Autodesk Inventor part; units mm, degrees
ref_plane "YZ Plane" through (0, 0, 0) normal (1, 0, 0) x (0, 1, 0)
ref_plane "XZ Plane" through (0, 0, 0) normal (0, 1, 0) x (-1, 0, 0)
ref_plane "XY Plane" through (0, 0, 0) normal (0, 0, 1) x (1, 0, 0)
sketch "Sketch1" plane through (0, 0, 0) normal (0, 1, 0) x (-1, 0, 0)
  line L0 (-43.3, -50.05) -> (43.3, -50.05)
  line L1 (43.3, -50.05) -> (43.3, 50.05)
  line L2 (43.3, 50.05) -> (-43.3, 50.05)
  line L3 (-43.3, 50.05) -> (-43.3, -50.05)
  line L4 (-43.3, -50.05) -> (43.3, 50.05) construction
  line L5 (43.3, -50.05) -> (-43.3, 50.05) construction
  point P0 (0, 0)
  dimension "d0" = 86.6
  dimension "d1" = 100.1
extrude "Extrusion1" add sketch "Sketch1" along normal blind 4.445
sketch "Sketch2" plane through (0, 4.445, 0) normal (0, 1, 0) x (1, 0, 0)
  line L0 (40.1, 46.85) -> (-40.1, 46.85)
  line L1 (-40.1, 46.85) -> (-40.1, -46.85)
  line L2 (-40.1, -46.85) -> (40.1, -46.85)
  line L3 (40.1, -46.85) -> (40.1, 46.85)
  line L4 (40.1, 46.85) -> (-40.1, -46.85) construction
  line L5 (-40.1, 46.85) -> (40.1, -46.85) construction
  line L6 (-43.3, 50.05) -> (-43.3, -50.05)
  line L7 (-43.3, -50.05) -> (43.3, -50.05)
  line L8 (43.3, 50.05) -> (-43.3, 50.05)
  line L9 (43.3, -50.05) -> (43.3, 50.05)
  line L10 (36.9, -43.65) -> (43.3, -50.05) construction
  line L11 (34.4431, -46.85) -> (40.4716, -52.8784)
  line L12 (46.1284, -47.2216) -> (40.1, -41.1931)
  arc A0 (40.4716, -52.8784) -> (46.1284, -47.2216) centre (43.3, -50.05) ccw
  circle A1 centre (43.3, -50.05) radius 1.375
  point P0 (0, 0)
  dimension "d4" = 3.2
  dimension "d5" = 3.2
  dimension "d22" = 8
  dimension "d23" = 2.75
extrude "Extrusion2" add sketch "Sketch2" along normal blind 49 contours L0 L1 L2 L11 L7 L6 L8 L9 L12 L3 | L12 L9 A1 L7 L11 L2 L3 | L9 L7 A1 picked at (42.4402, -49.7491)
sketch "Sketch4" plane through (0, 0, 0) normal (0, -1, 0) x (1, 0, 0)
  line L0 (41.7906, 48.7379) -> (44.8094, 51.3621) construction
  line L1 (43.3, 50.05) -> (43.3, -50.05)
  line L2 (43.3, 44.7499) -> (47.4337, 48.3433)
  line L3 (42.1852, 54.381) -> (39.1663, 51.7567)
  arc A0 (39.1663, 51.7567) -> (38.0119, 50.05) centre (41.7906, 48.7379) ccw
  arc A1 (47.4337, 48.3433) -> (42.1852, 54.381) centre (44.8094, 51.3621) ccw
  line L4 (-43.3, 50.05) -> (43.3, 50.05)
  line L5 (38.0119, 50.05) -> (43.3, 50.05)
  line L6 (43.3, 50.05) -> (43.3, 44.7499)
  circle A2 centre (44.8094, 51.3621) radius 1.985
  line L7 (0, 50.05) -> (0, -50.05) construction
  line L8 (43.3, -50.05) -> (-43.3, -50.05) construction
  line L9 (43.3, 0) -> (-33.3, 0) construction
  line L10 (43.3, -50.05) -> (43.3, 50.05)
  line L11 (43.3, -44.7499) -> (47.4337, -48.3433)
  line L12 (42.1852, -54.381) -> (39.1663, -51.7567)
  arc A3 (38.0119, -50.05) -> (39.1663, -51.7567) centre (41.7906, -48.7379) ccw
  arc A4 (42.1852, -54.381) -> (47.4337, -48.3433) centre (44.8094, -51.3621) ccw
  line L13 (-43.3, -50.05) -> (43.3, -50.05)
  circle A5 centre (44.8094, -51.3621) radius 1.985
  line L14 (-43.3, 50.05) -> (-43.3, -50.05)
  line L15 (-43.3, 44.7499) -> (-47.4337, 48.3433)
  line L16 (-42.1852, 54.381) -> (-39.1663, 51.7567)
  arc A6 (-38.0119, 50.05) -> (-39.1663, 51.7567) centre (-41.7906, 48.7379) ccw
  arc A7 (-42.1852, 54.381) -> (-47.4337, 48.3433) centre (-44.8094, 51.3621) ccw
  line L17 (-38.0119, 50.05) -> (-43.3, 50.05)
  circle A8 centre (-44.8094, 51.3621) radius 1.985
  arc A9 (-47.4337, -48.3433) -> (-42.1852, -54.381) centre (-44.8094, -51.3621) ccw
  line L18 (-43.3, -44.7499) -> (-47.4337, -48.3433)
  line L19 (-42.1852, -54.381) -> (-39.1663, -51.7567)
  arc A10 (-39.1663, -51.7567) -> (-38.0119, -50.05) centre (-41.7906, -48.7379) ccw
  circle A11 centre (-44.8094, -51.3621) radius 1.985
  line L20 (-38.0119, -50.05) -> (-43.3, -50.05)
  line L21 (-43.3, -50.05) -> (-43.3, 50.05)
  point P0 (0, 0)
  point P1 (-38.0119, -50.05)
  point P2 (-43.3, -44.7499)
  point P3 (-38.0119, 50.05)
  point P4 (43.3, -44.7499)
  point P5 (43.3, -50.05)
  dimension "d24" = 2
  dimension "d25" = 8
  dimension "d26" = 131
  dimension "d27" = 3.97
extrude "Extrusion4" add sketch "Sketch4" against normal up to surface (53.445 mm away) contours L4 A0 L3 A1 L2 L1 | L11 A4 L12 A3 L13 L1 | L4 L14 L15 A7 L16 A6 | A10 L19 A9 L18 L14 L13
fillet "Fillet2" radius 2 4 edges at (40.1, 28.945, -46.85) (-40.1, 28.945, -46.85) (-40.1, 28.945, 46.85) (40.1, 28.945, 46.85)
sketch "Sketch14" plane through (0, 4.445, 0) normal (0, 1, 0) x (1, 0, 0)
  circle A0 centre (36.6, -34.85) radius 3.7
  circle A1 centre (36.6, -34.85) radius 1.985
  line L0 (38.1, -46.85) -> (-38.1, -46.85)
  line L1 (40.1, 44.85) -> (40.1, -44.85)
  line L2 (-38.1, -46.85) -> (38.1, -46.85) construction
  line L3 (0, -46.85) -> (0, 50.05) construction
  line L4 (38.0119, 50.05) -> (-38.0119, 50.05) construction
  circle A2 centre (36.6, 23.15) radius 3.7
  circle A3 centre (36.6, 23.15) radius 1.985
  line L5 (-40.1, 44.85) -> (-40.1, -44.85) construction
  line L6 (-40.1, 0) -> (40.1, 0) construction
  line L7 (40.1, -44.85) -> (40.1, 44.85) construction
  circle A4 centre (-12.4, -34.85) radius 3.7
  circle A5 centre (-12.4, -34.85) radius 1.985
  circle A6 centre (-12.4, 23.15) radius 1.985
  circle A7 centre (-12.4, 23.15) radius 3.7
  point P0 (0, 0)
  dimension "d114" = 7.4
  dimension "d115" = 3.97
  dimension "d116" = 12
  dimension "d117" = 3.5
  dimension "d120" = 58
  dimension "d127" = 49
sketch "Sketch15" plane through (0, 4.445, 0) normal (0, 1, 0) x (1, 0, 0)
  point P0 (0, 0)
extrude "Extrusion10" add sketch "Sketch14" along normal blind 6
sketch "Sketch16" plane through (43.3, 0, 44.7499) normal (1, 0, 0) x (0, 0, -1)
  line L0 (12.9515, 13.2621) -> (12.9515, 13.455)
  line L1 (20.9323, 13.455) -> (20.9323, 13.2621)
  line L2 (13.9419, 14.5004) -> (19.9419, 14.5004)
  line L3 (88.3241, 11.975) -> (9.3999, 11.975)
  line L4 (22.9323, 9.975) -> (10.9515, 9.975)
  line L5 (10.9515, 9.975) -> (10.9515, 19.0004)
  line L6 (10.9515, 19.0004) -> (22.9323, 19.0004)
  line L7 (22.9323, 19.0004) -> (22.9323, 9.975)
  line L8 (30.8419, 17.055) -> (30.8419, 14.5766)
  line L9 (45.8419, 14.5766) -> (45.8419, 17.055)
  line L10 (45.0419, 17.855) -> (31.6419, 17.855)
  line L11 (47.8419, 10.975) -> (28.8419, 10.975)
  line L12 (28.8419, 10.975) -> (28.8419, 19.855)
  line L13 (28.8419, 19.855) -> (47.8419, 19.855)
  line L14 (47.8419, 19.855) -> (47.8419, 10.975)
  line L15 (56.4419, 17.775) -> (56.4419, 11.775)
  line L16 (63.4419, 11.775) -> (63.4419, 17.775)
  line L17 (63.4419, 17.775) -> (59.9419, 17.775)
  line L18 (59.9419, 17.775) -> (56.4419, 17.775)
  line L19 (64.9419, 10.975) -> (54.9419, 10.975)
  line L20 (54.9419, 10.975) -> (54.9419, 19.275)
  line L21 (54.9419, 19.275) -> (64.9419, 19.275)
  line L22 (64.9419, 19.275) -> (64.9419, 10.975)
  point P0 (44.7499, 0)
  dimension "d134" = 4.5
  dimension "d135" = 2
  dimension "d136" = 2
  dimension "d137" = 2
  dimension "d138" = 2
  dimension "d139" = 1
  dimension "d140" = 2
  dimension "d141" = 2
  dimension "d142" = 1
  dimension "d143" = 1.5
  dimension "d144" = 1.5
  dimension "d145" = 1.5
extrude "Extrusion11" cut sketch "Sketch16" against normal up to surface (3.2 mm away)
sketch "Sketch17" plane through (38.0119, 0, -50.05) normal (0, 0, -1) x (-1, 0, 0)
  line L0 (16.1912, 11.975) -> (16.1912, 25.475)
  line L1 (0.3112, 11.975) -> (0.3112, 25.475)
  line L2 (0.3112, 25.475) -> (16.1912, 25.475)
  line L3 (50.9119, 11.975) -> (0.9119, 11.975)
  line L4 (16.4912, 11.725) -> (0.0112, 11.725)
  line L5 (0.0112, 11.725) -> (0.0112, 25.725)
  line L6 (0.0112, 25.725) -> (16.4912, 25.725)
  line L7 (16.4912, 25.725) -> (16.4912, 11.725)
  line L8 (19.4512, 18.7546) -> (19.4512, 21.7546)
  line L9 (34.5512, 21.7546) -> (34.5512, 18.7546)
  line L10 (24.0012, 27.465) -> (30.0012, 27.465)
  line L11 (35.2512, 11.225) -> (18.7512, 11.225)
  line L12 (18.7512, 11.225) -> (18.7512, 28.465)
  line L13 (18.7512, 28.465) -> (35.2512, 28.465)
  line L14 (35.2512, 28.465) -> (35.2512, 11.225)
  line L15 (37.4512, 18.7546) -> (37.4512, 21.7546)
  line L16 (52.5512, 21.7546) -> (52.5512, 18.7546)
  line L17 (42.0012, 27.465) -> (48.0012, 27.465)
  line L18 (53.2512, 11.225) -> (36.7512, 11.225)
  line L19 (36.7512, 11.225) -> (36.7512, 28.465)
  line L20 (36.7512, 28.465) -> (53.2512, 28.465)
  line L21 (53.2512, 28.465) -> (53.2512, 11.225)
  point P0 (38.0119, 0)
  point P1 (18.7512, 11.975)
  point P2 (35.2512, 11.975)
  dimension "d148" = 0.3
  dimension "d149" = 0.3
  dimension "d150" = 0.25
  dimension "d151" = 0.25
  dimension "d154" = 0.7
  dimension "d155" = 0.7
  dimension "d156" = 1
  dimension "d157" = 0.75
  dimension "d158" = 1
  dimension "d159" = 0.7
  dimension "d160" = 0.7
  dimension "d161" = 0.75
extrude "Extrusion12" cut sketch "Sketch17" against normal up to surface (3.2 mm away)
sketch "Sketch19" plane through (-43.3, 0, -44.7499) normal (-1, 0, 0) x (0, 0, 1)
  circle A0 centre (20, 25) radius 9.6
  line L0 (0, 53.445) -> (0, 0)
  line L1 (0, 0) -> (89.4999, 0)
  point P0 (44.7499, 0)
  dimension "d162" = 19.2
  dimension "d163" = 20
  dimension "d164" = 25
extrude "Extrusion13" cut sketch "Sketch19" against normal up to surface (3.2 mm away)
sketch "Sketch23" plane through (-43.3, 0, -44.7499) normal (-1, 0, 0) x (0, 0, 1)
  line L0 (52.1999, 9.1) -> (79.4999, 9.1)
  line L1 (79.4999, 9.1) -> (79.4999, 36.9)
  line L2 (79.4999, 36.9) -> (52.1999, 36.9)
  line L3 (52.1999, 36.9) -> (52.1999, 9.1)
  line L4 (89.4999, 0) -> (89.4999, 53.445)
  line L5 (0, 0) -> (89.4999, 0)
  circle A0 centre (54.1999, 34.9) radius 1
  line L6 (65.8499, 36.9) -> (65.8499, 9.1) construction
  line L7 (52.1999, 23) -> (79.4999, 23) construction
  circle A1 centre (77.4999, 34.9) radius 1
  circle A2 centre (54.1999, 11.1) radius 1
  circle A3 centre (77.4999, 11.1) radius 1
  line L8 (78.8499, 19.53) -> (52.8499, 19.53)
  line L9 (52.8499, 19.53) -> (52.8499, 30.53)
  line L10 (52.8499, 30.53) -> (78.8499, 30.53)
  line L11 (78.8499, 30.53) -> (78.8499, 19.53)
  line L12 (78.8499, 19.53) -> (52.8499, 30.53) construction
  line L13 (52.8499, 19.53) -> (78.8499, 30.53) construction
  line L14 (79.1999, 13.37) -> (52.4999, 13.37)
  line L15 (52.4999, 13.37) -> (52.4999, 32.63)
  line L16 (52.4999, 32.63) -> (79.1999, 32.63)
  line L17 (79.1999, 32.63) -> (79.1999, 13.37)
  line L18 (79.1999, 13.37) -> (52.4999, 32.63) construction
  line L19 (52.4999, 13.37) -> (79.1999, 32.63) construction
  point P0 (44.7499, 0)
  point P1 (65.8499, 25.03)
  point P2 (65.8499, 23)
  dimension "d208" = 27.3
  dimension "d209" = 27.8
  dimension "d210" = 10
  dimension "d212" = 2
  dimension "d213" = 2
  dimension "d214" = 2
  dimension "d215" = 26
  dimension "d216" = 11
  dimension "d217" = 6.37
  dimension "d218" = 26.7
  dimension "d219" = 19.26
  dimension "d220" = 4.27
  dimension "d223" = 23
extrude "Extrusion17" cut sketch "Sketch23" against normal up to surface (3.2 mm away) contours A0 | A1 | A2 | A3 | L8 L9 L10 L11
properties part number "_3DPrint"
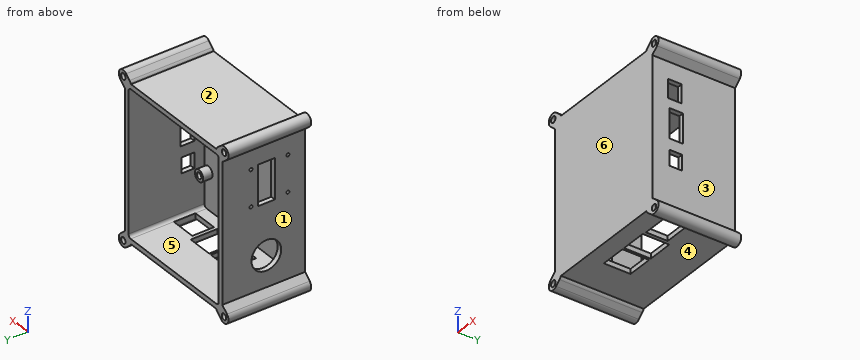
Part model, mm, in its own coordinate system. Face numbers are marked on the shaded views. A direction names the side the tool comes from. Round coordinates to 2 decimals unless told otherwise and drop trailing zeros. Write each loop counter-clockwise with the first axis right and the second up, starting at its lowest first coordinate (ties: lowest second). Pieces come first, ordered by that corner, then holes.
Item 1: Cut at A-A, the plane x = -12.4. Give the cut face in (y, z) (3 decimals).
Results:
outline: (0, -50.05) - (11.225, -50.05) - (11.225, -46.85) - (4.445, -46.85) - (4.445, -26.85) - (10.445, -26.85) - (10.445, -25.135) - (4.445, -25.135) - (4.445, -21.165) - (10.445, -21.165) - (10.445, -19.45) - (4.445, -19.45) - (4.445, 31.15) - (10.445, 31.15) - (10.445, 32.865) - (4.445, 32.865) - (4.445, 36.835) - (10.445, 36.835) - (10.445, 38.55) - (4.445, 38.55) - (4.445, 46.85) - (53.445, 46.85) - (53.445, 50.05) - (0, 50.05) - close; (28.465, -50.05) - (53.445, -50.05) - (53.445, -46.85) - (28.465, -46.85) - close
Item 2: Cut at C-C, the plane x = 14. Give the cut face in (y, z) (3 decimals).
Results:
outline: (0, -50.05) - (11.225, -50.05) - (11.225, -46.85) - (4.445, -46.85) - (4.445, 46.85) - (53.445, 46.85) - (53.445, 50.05) - (0, 50.05) - close; (28.465, -50.05) - (53.445, -50.05) - (53.445, -46.85) - (28.465, -46.85) - close
Item 3: Drop flat-ended pins along their axis: pin 1 Ø5 at (y, z) = (18.5, -17.5) entering from +X; pin 2 Ø4 at (x, y) = (37, 10.5) entering from -Z; pin 3 Ø1.6 at (x, y) = (-42.5, 26) entering from -Z. Give the stop position or say it passes through.
Results:
pin 1: stops at x = 43.3
pin 2: stops at z = -51.6
pin 3: stops at z = -55.07
Item 4: Cut at B-B, the plane x = -23. Give the cut face in (y, z) (3 decimals), plus the area to 3 significant figures.
Results:
outline: (0, -50.05) - (53.445, -50.05) - (53.445, -46.85) - (4.445, -46.85) - (4.445, 46.85) - (53.445, 46.85) - (53.445, 50.05) - (0, 50.05) - close
area: 759 mm2
Item 5: Cut at D-D, the plane y = 42. Count the separate pieces of the cut face and the enclosed holes in it, plus the area to 3 significant figures.
Results:
separate pieces: 1
enclosed holes: 5
area: 1,330 mm2
Item 6: Two-plate mould, pull along X, no slides. Class the marked faces 1, 2 and 3: +X half, -X half, draft (parallel to the pull), parting line (faces both ways), or undercut.
Results:
face 1: -X half
face 2: undercut
face 3: +X half
Item 7: Probe L1, parallel to X at y = 8.65, z = 34.85 (3 decimals); L2, parallel to X at y = 33, z = -3; L3, parallel to Z at x = 11.5, y = 51. List the from-to ranges inside material, lowest first.
Results:
L1: x = -43.3 to -40.1, -16.1 to -14.385, -10.415 to -8.7, 32.9 to 34.615, 38.585 to 43.3
L2: x = -43.3 to -40.1, 40.1 to 43.3
L3: z = -50.05 to -46.85, 46.85 to 50.05
Item 8: Which spindle directions (+Z, -Z, +X, -X, +Y, -Y) get a long thin tool onto all of the face, cutting with end or side? Do the marked faces 4, 5 and 6. Say none if no direction does.
Results:
face 4: -Z, +Y, -Y
face 5: +Y
face 6: +Z, -Z, +X, -X, -Y
